Geometry check sheet. Reference: the model listing, model coordinates, mm. Face numbers are marked on the shaded views. A direction names the side the tool comes from. Give positions to 0.01 mm unless a question says otherwise; leave off trailing zeros. Loops run counter-clockwise (first coordinate to the right, second up) from the corner with the lowest first, then second, coordinate; pieces in that order, holes last. Notation, with made-up numbers: (85.5, 6.5) -> (110.5, 6.5) arc R3 ccw to (110.5, 10.5) -> close; hole circle Ø4 at (31, 40). An arc over 180 degrees is marked (long way). One line per item, written item: value. Start each with the question number.
(1) Sectioned sample at D-D, the plane z = -7. Record the cut outline in (x, y), then the cut area to 3 significant figures.
(2) Gauge pin test, flat ends, axial feed: pin 1 Ø4 at (x, z) = (-4.05, -3.07) entering from +Y; pin 2 Ø2 at (x, y) = (3, 10) entering from +Z; pin 3 Ø10 at (y, z) = (9.5, 14) entering from -X; pin 4 Ø4 at (x, z) = (5.6, 0) entering from -Y. Record the tip position at first contact, or that the pin passes through.
(3) Sectioned sample at A-A, the plane z = 0. Record the cut outline in (x, y) (3 decimals).
(4) Tool access check on the marked faces 1, 2 and 3. Record the directions out of +Z, -Z, +X, -X, +Y, -Y that give a thin tool (end or side, any length) a straight path to the whole face; none if there is none.
(5) Scan lines: line 1 along Z through (x, y) = (0, 9.5) (3 decimals); line 2 along Z through (x, y) = (-4.5, 15.25); line 3 along Z through (x, y) = (4.5, 15.5). Record each from-to range of solid material in increasing order. Write a range as from..to.
(6) Sectioned sample at C-C, the plane y = 22.25. Record the cut outline in (x, z) (3 decimals).
(7) Sectioned sample at B-B, the plane x = -0.5. Record the cut outline in (y, z), then the cut area to 3 significant figures.
(8) Draft check along Z on the marked faces 4, 5 and 6. Enter one of: pulls with the +Z half, pulls with the -Z half, needs draft (parallel to the pull), parting line crosses it, or undercut.
from build123d import *

# Parameters (mm, degrees)
F0_R     = 19.685
F1_DEPTH = 16.51
F2_R     = 8.636
F3_DEPTH = 13.208
F4_R     = 3.175
F5_DEPTH = 8.89
F6_R     = 1.273629
F7_DEPTH = 25.4


with BuildPart() as f1:
    # F0 (on Front) → F1 (new body)
    with BuildSketch(Plane.XZ):
        Circle(F0_R)
    extrude(amount=-F1_DEPTH)

    # F2 (on Front) → F3 (cut)
    with BuildSketch(Plane.XZ):
        Circle(F2_R)
    extrude(amount=-F3_DEPTH, mode=Mode.SUBTRACT)

    # F4 (on face) → F5 (join)
    with BuildSketch(Plane(origin=(0, 16.51, 0), x_dir=(-1, 0, 0), z_dir=(0, 1, 0))):
        Circle(F4_R)
    extrude(amount=F5_DEPTH)

    # F6 (on face) → F7 (cut)
    with BuildSketch(Plane.XZ.offset(-13.208)):
        with BuildLine():
            ThreePointArc((5.419761, 3.070403), (3.609433, 4.371419), (2.953539, 2.240753))
            ThreePointArc((2.953539, 2.240753), (4.484769, 1.769387), (5.419761, 3.070403))
        make_face()
        with BuildLine():
            ThreePointArc((6.868104, 0), (5.598104, 1.27), (4.328104, 0))
            ThreePointArc((4.328104, 0), (5.598104, -1.27), (6.868104, 0))
        make_face()
        with BuildLine():
            ThreePointArc((5.317101, -3.070403), (4.452036, -1.866689), (3.035326, -2.302802))
            ThreePointArc((3.035326, -2.302802), (3.642166, -4.274117), (5.317101, -3.070403))
        make_face()
        with BuildLine():
            ThreePointArc((-2.777101, -3.070403), (-2.843387, -2.665467), (-3.035326, -2.302802))
            ThreePointArc((-3.035326, -2.302802), (-5.250815, -3.475338), (-2.777101, -3.070403))
        make_face()
        with BuildLine():
            ThreePointArc((1.27, -5.08), (0.898026, -4.181974), (0, -3.81))
            ThreePointArc((0, -3.81), (-0.898026, -5.978026), (1.27, -5.08))
        make_face()
        with Locations((-4.561896, 0)):
            Circle(F6_R)
        with BuildLine():
            ThreePointArc((-2.777101, 3.070403), (-5.250815, 3.475338), (-3.035326, 2.302802))
            ThreePointArc((-3.035326, 2.302802), (-2.843387, 2.665467), (-2.777101, 3.070403))
        make_face()
        with BuildLine():
            ThreePointArc((1.27, 5.08), (-0.898026, 5.978026), (0, 3.81))
            ThreePointArc((0, 3.81), (0.898026, 4.181974), (1.27, 5.08))
        make_face()
    extrude(amount=-F7_DEPTH, mode=Mode.SUBTRACT)


solid = f1.part
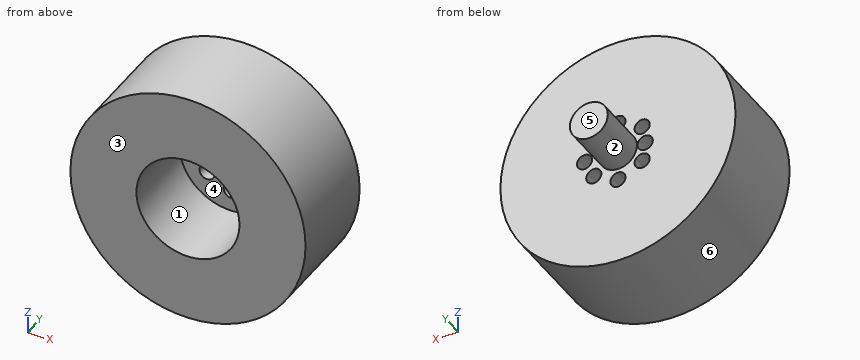
Calculated:
1. outline: (-18.4, 0) -> (-5.06, 0) -> (-5.06, 13.21) -> (5.06, 13.21) -> (5.06, 0) -> (18.4, 0) -> (18.4, 16.51) -> (-18.4, 16.51) -> close
1. area: 474 mm2
2. pin 1: stops at y = 25.4
2. pin 2: stops at z = 19.58
2. pin 3: stops at x = -17.51
2. pin 4: stops at y = 13.21
3. outline: (-19.685, 0) -> (-8.636, 0) -> (-8.636, 13.208) -> (-5.836, 13.208) -> (-5.836, 16.51) -> (-19.685, 16.51) -> close; (-3.288, 13.208) -> (4.328, 13.208) -> (4.328, 16.51) -> (3.175, 16.51) -> (3.175, 25.4) -> (-3.175, 25.4) -> (-3.175, 16.51) -> (-3.288, 16.51) -> close; (6.868, 13.208) -> (8.636, 13.208) -> (8.636, 0) -> (19.685, 0) -> (19.685, 16.51) -> (6.868, 16.51) -> close
4. face 1: -Y
4. face 2: +Y
4. face 3: +Z, -Z, +X, -X, -Y
5. line 1: z = -19.685..-8.636, 8.636..19.685
5. line 2: z = -19.16..-4.26, -1.88..-1.27, 1.27..1.88, 4.26..19.16
5. line 3: z = -19.16..-4.26, -1.88..-0.64, 0.64..1.77, 4.37..19.16
6. outline: circle Ø6.35 at (0, 0)
7. outline: (0, -19.68) -> (16.51, -19.68) -> (16.51, -6.25) -> (13.21, -6.25) -> (13.21, -8.62) -> (0, -8.62) -> close; (0, 8.62) -> (13.21, 8.62) -> (13.21, 6.25) -> (16.51, 6.25) -> (16.51, 19.68) -> (0, 19.68) -> close; (13.21, -3.91) -> (16.51, -3.91) -> (16.51, -3.14) -> (25.4, -3.14) -> (25.4, 3.14) -> (16.51, 3.14) -> (16.51, 3.91) -> (13.21, 3.91) -> close
7. area: 462 mm2
8. face 4: undercut
8. face 5: needs draft
8. face 6: parting line crosses it
